```python
from build123d import *

# Parameters (mm, degrees)
SKETCH1_W               = 25.4
SKETCH1_H               = 25.4
SKETCH1_W_2             = 21.4
SKETCH1_H_2             = 21.4
BOSS_EXTRUDE1_DEPTH     = 675.4
SKETCH3_R               = 3
CUT_EXTRUDE1_DEPTH      = 650
CUT_EXTRUDE2_DEPTH      = 676.996752951
CUT_EXTRUDE2_DEPTH_BACK = 676.996752951
SKETCH4_R               = 2


with BuildPart() as part:
    # Sketch1 → Boss-Extrude1 (new body)
    with BuildSketch(Plane.XY):
        Rectangle(SKETCH1_W, SKETCH1_H)
        Rectangle(SKETCH1_W_2, SKETCH1_H_2, mode=Mode.SUBTRACT)
    extrude(amount=BOSS_EXTRUDE1_DEPTH)

    # Sketch3 → Cut-Extrude1 (cut)
    with BuildSketch(Plane(origin=(0, 12.7, 0), x_dir=(1, 0, 0), z_dir=(0, 1, 0))):
        with Locations(Location((0, -662.7, 0), (0, 0, 180))):
            Circle(SKETCH3_R)
        with Locations(Location((0, -612.7, 0), (0, 0, 180))):
            Circle(SKETCH3_R)
        with Locations(Location((0, -562.7, 0), (0, 0, 180))):
            Circle(SKETCH3_R)
        with Locations(Location((0, -512.7, 0), (0, 0, 180))):
            Circle(SKETCH3_R)
        with Locations(Location((0, -462.7, 0), (0, 0, 180))):
            Circle(SKETCH3_R)
        with Locations(Location((0, -412.7, 0), (0, 0, 180))):
            Circle(SKETCH3_R)
        with Locations(Location((0, -362.7, 0), (0, 0, 180))):
            Circle(SKETCH3_R)
        with Locations(Location((0, -312.7, 0), (0, 0, 180))):
            Circle(SKETCH3_R)
        with Locations(Location((0, -262.7, 0), (0, 0, 180))):
            Circle(SKETCH3_R)
        with Locations(Location((0, -212.7, 0), (0, 0, 180))):
            Circle(SKETCH3_R)
        with Locations(Location((0, -162.7, 0), (0, 0, 180))):
            Circle(SKETCH3_R)
        with Locations(Location((0, -112.7, 0), (0, 0, 180))):
            Circle(SKETCH3_R)
        with Locations(Location((0, -62.7, 0), (0, 0, 180))):
            Circle(SKETCH3_R)
        with Locations(Location((0, -12.7, 0), (0, 0, 180))):
            Circle(SKETCH3_R)
    extrude(amount=-CUT_EXTRUDE1_DEPTH, mode=Mode.SUBTRACT)

    # Sketch4 → Cut-Extrude2 (cut, two sides: drawn at the far end of the back side and taken through both)
    with BuildSketch(Plane(origin=(12.7, 0, 0), x_dir=(0, 0, -1), z_dir=(1, 0, 0)).offset(-CUT_EXTRUDE2_DEPTH_BACK)):
        with Locations((-44.1, 0)):
            Circle(SKETCH4_R)
        with Locations((-32.1, 0)):
            Circle(SKETCH4_R)
        with Locations((-117.5, 0)):
            Circle(SKETCH4_R)
        with Locations((-129.5, 0)):
            Circle(SKETCH4_R)
        with Locations(Location((-643.3, 0, 0), (0, 0, 90))):
            Circle(SKETCH4_R)
        with Locations(Location((-631.3, 0, 0), (0, 0, 90))):
            Circle(SKETCH4_R)
        with Locations(Location((-557.9, 0, 0), (0, 0, 90))):
            Circle(SKETCH4_R)
        with Locations(Location((-545.9, 0, 0), (0, 0, 90))):
            Circle(SKETCH4_R)
    extrude(amount=CUT_EXTRUDE2_DEPTH + CUT_EXTRUDE2_DEPTH_BACK, mode=Mode.SUBTRACT)


solid = part.part
```
The listing builds one solid part. Answer for the finished solid, in the listing's coordinates (mm). A direction names the side the tool comes from. Coordinates: 2 decimals unless noted, no trailing zeros. Write each loop counter-clockwise with the first axis right and the second up, starting at its lowest first coordinate (ties: lowest second). Pieces come first, ordered by that corner, then holes.
Q1. Section B-B, the plane z = 321.5 is taken. Write down the section's boundary in (x, y).
Returned:
outline: (-12.7, -12.7) - (12.7, -12.7) - (12.7, 12.7) - (-12.7, 12.7) - close; hole (-10.7, -10.7) - (10.7, -10.7) - (10.7, 10.7) - (-10.7, 10.7) - close
Q2. Section A-A, the plane y = -6 is taken. Write down the section's boundary in (x, z), then the cut area to 3 significant figures.
Returned:
outline: (-12.7, 0) - (-10.7, 0) - (-10.7, 675.4) - (-12.7, 675.4) - close; (10.7, 0) - (12.7, 0) - (12.7, 675.4) - (10.7, 675.4) - close
area: 2,700 mm2
Q3. Find the intervals of material crossed by line 1 along X through (y, z) = (-8.5, 149); line 2 along Y through (x, z) = (11.2, 631.3), in increasing order.
Returned:
line 1: x = -12.7 to -10.7, 10.7 to 12.7
line 2: y = -12.7 to -2, 2 to 12.7
Q4. The mould has two halves that part along X. Classify faces 3 (the flat face through (-12.7, 0, 333)), 4 (the flat face through (0, 10.7, 333)), 5 (the flat face through (0, 12.7, 333)): released by +X, released by -X, zero draft, split by the parting line, or undercut.
Returned:
face 3: released by -X
face 4: undercut
face 5: zero draft
Q5. Which of the six approach directions +Z, -Z, +X, -X, +Y, -Y give full straight-line access (tool end or side, diameter ignored) to faces 1 (the flat face through (10.7, 0, 333)), 2 (the flat face through (0, -12.7, 333))?
Returned:
face 1: +Z, -Z
face 2: +Z, -Z, +X, -X, -Y
